Autodesk Inventor part; units mm, degrees
ref_plane "YZ Plane" through (0, 0, 0) normal (1, 0, 0) x (0, 1, 0)
ref_plane "XZ Plane" through (0, 0, 0) normal (0, 1, 0) x (-1, 0, 0)
ref_plane "XY Plane" through (0, 0, 0) normal (0, 0, 1) x (1, 0, 0)
sketch "Sketch1" plane through (0, 0, 0) normal (0, 1, 0) x (-1, 0, 0)
  line L0 (3.7362, 151.865) -> (-2.2638, 151.865)
  line L1 (-2.2638, 151.865) -> (-2.2638, -8.135)
  line L2 (-2.2638, -8.135) -> (3.7362, -8.135)
  line L3 (3.7362, -8.135) -> (3.7362, 151.865)
  point P0 (0, 0)
  dimension "d0" = 6
  dimension "d1" = 160
extrude "Extrusion1" add sketch "Sketch1" along normal blind 20
sketch "Sketch2" plane through (-3.7362, 0, -8.135) normal (-1, 0, 0) x (0, 0, 1)
  line L0 (160, 20) -> (0, 20)
  line L1 (15, 20) -> (145, 20)
  line L2 (145, 20) -> (145, 0)
  line L3 (145, 0) -> (15, 0)
  line L4 (15, 0) -> (15, 20)
  line L5 (0, 0) -> (0, 20)
  line L6 (160, 0) -> (160, 20)
  point P0 (8.135, 0)
  dimension "d4" = 15
  dimension "d5" = 15
  dimension "d6" = 20
extrude "Extrusion2" add sketch "Sketch2" along normal blind 50
sketch "Sketch3" plane through (0, 20, 0) normal (0, 1, 0) x (1, 0, 0)
  line L0 (-3.7362, -136.865) -> (-53.7362, -136.865)
  line L1 (-53.7362, -6.865) -> (-23.7362, -6.865)
  line L2 (-23.7362, -6.865) -> (-23.7362, -136.865)
  line L3 (-23.7362, -136.865) -> (-53.7362, -136.865)
  line L4 (-53.7362, -136.865) -> (-53.7362, -6.865)
  point P0 (0, 0)
  dimension "d9" = 30
extrude "Extrusion3" add sketch "Sketch3" along normal blind 100
sketch "Sketch4" plane through (-3.7362, 0, 6.865) normal (0, 0, -1) x (-1, 0, 0)
  line L0 (50, 0) -> (66, 0)
  line L1 (66, 0) -> (66, 50)
  line L2 (66, 50) -> (50, 50)
  line L3 (50, 50) -> (50, 0)
  point P0 (-3.7362, 0)
  dimension "d12" = 16
  dimension "d13" = 50
extrude "Extrusion4" add sketch "Sketch4" against normal blind 50
sketch "Sketch6" plane through (0, 20, 0) normal (0, 1, 0) x (1, 0, 0)
  line L0 (-23.7362, -6.865) -> (-23.7362, -136.865)
  line L1 (-3.7362, -129.865) -> (-23.7362, -129.865)
  line L2 (-23.7362, -129.865) -> (-23.7362, -13.865)
  line L3 (-23.7362, -13.865) -> (-3.7362, -13.865)
  line L4 (-3.7362, -13.865) -> (-3.7362, -129.865)
  line L5 (-3.7362, -136.865) -> (-23.7362, -136.865)
  line L6 (2.2638, -151.865) -> (2.2638, 8.135)
  line L7 (-3.7362, -6.865) -> (-23.7362, -6.865)
  point P0 (0, 0)
  dimension "d16" = 7
  dimension "d17" = 6
  dimension "d18" = 7
extrude "Extrusion5" cut sketch "Sketch6" against normal blind 50
fillet "Fillet1" radius 5 4 edges at (-23.7362, 20, 133.365) (-23.7362, 20, 10.365) (-23.7362, 10, 129.865) (-23.7362, 10, 13.865)
fillet "Fillet2" radius 5 4 edges at (-3.7362, 10, 129.865) (-3.7362, 10, 13.865) (-3.7362, 10, 6.865) (-3.7362, 10, 136.865)
properties part number "E_box"
Model file for the job. Use its own axes, mm. A direction names the side the tool comes from. Round coordinates to 2 decimals unless told otherwise and drop trailing zeros. Order: outer loops, then holes, each group sorted by start corner. A loop starts at its lowest first (then second) coordinate and runs counter-clockwise, first axis right, second up. Notation, with made-up numbers: M 76,46 L 117,46 A23 cw 117,64 Z; hole C 12,41 d10. An arc over 180 degrees is marked long. Write each question's results on one line, items separated by ' | '. Start each with the question number.
(1) Probe probe 1 along X at (y, z) = (58.5, 53); probe 2 along X at (y, z) = (26, 21.5); probe 3 along Y at (x, z) = (-60, 39.5). List the from-to ranges inside material, lowest first. Write a range as from..to.
(2) Saw through at A-A, the plane x = -14. Give the cut face in (y, z) (3 decimals).
(3) Which spindle directions (+Z, -Z, +X, -X, +Y, -Y) get a long thin tool onto all of the face, cutting with end or side? Do faces 1 (the face through (-3, 20, 60)), 2 (the face through (-39, 48, 6.865)), 3 (the face through (-14, 10, 13.865)), 4 (the face through (-62, 50, 32)), 5 (the face through (-36, 59, 136.865)). Say none if no direction does.
(4) Saw through at D-D, the plane z = 134. Give the cut face in (x, y), then the cut area to 3 significant figures.
(5) Two-plate mould, pull along Z, no slides. Class faces 6 (the face through (-3.736, 10, 71)), 7 (the face through (-62, 25, 56.865)), 8 (the face through (-22.31, 21.504, 11.616)): pulls with the +Z half, pulls with the -Z half, needs draft (parallel to the pull), parting line crosses it, or undercut.
(6) Saw through at B-B, the plane z = 73. Give the cut face in (x, y).
(7) Saw through at C-C, the plane y = 30.5. Give the cut face in (x, z) (3 decimals), then the cut area to 3 significant figures.
(8) Drop flat-ended pins along their axis: pin 1 (5 mm diameter, centred on y = 9.5, z = 144.5, fed in from -X); pin 2 (11 mm diameter, centred on y = 8, z = -1, fed in from -X); pin 3 (23 mm diameter, centred on x = -5, z = 52, fed in from +Y); pin 4 (3 mm diameter, centred on x = -17, z = 127, fed in from +Y). Give the stop position or say it passes through.
Established:
1) probe 1: x = -53.74..-23.74 | probe 2: x = -69.74..-23.74 | probe 3: y = 0..50
2) outline: M 0,6.865 L 20,6.865 L 20,13.865 L 0,13.865 Z; M 0,129.865 L 20,129.865 L 20,136.865 L 0,136.865 Z
3) face 1: +Z, -Z, +X, +Y | face 2: -Z, -X, +Y, -Y | face 3: +Y, -Y | face 4: +Z, -Z, -X, +Y | face 5: +Z, -X, +Y, -Y
4) outline: M -53.74,0 L 2.26,0 L 2.26,20 L -18.74,20 A5 cw -23.74,25 L -23.74,120 L -53.74,120 Z | area: 4,130 mm^2
5) face 6: undercut | face 7: pulls with the +Z half | face 8: needs draft
6) outline: M -53.74,0 L -23.74,0 L -23.74,120 L -53.74,120 Z; M -3.74,0 L 2.26,0 L 2.26,20 L -3.74,20 Z
7) outline: M -69.736,6.865 L -23.736,6.865 L -23.736,136.865 L -53.736,136.865 L -53.736,56.865 L -69.736,56.865 Z | area: 4,700 mm^2
8) pin 1: stops at x = -3.74 | pin 2: stops at x = -4.49 | pin 3: stops at y = 20 | pin 4: passes through
